Check sheet for the drawn part. Datum: minimum x, y, z corner. Units: mm. A direction names the side the tool comes from. Give positions to 0.01 mm unless a question says otherwise; leave off trailing zeros. Loops run counter-clockwise (first coordinate to the right, second up) from the corner with the lowest first, then second, coordinate; pieces in that order, holes last. Notation, with made-up numbers: (-10.75, -2.5) - (22.25, -2.5) arc R26 cw to (22.25, 19.5) - close; hole circle Ø8 at (84, 73.25). An arc over 180 degrees is marked (long way). Answer in a Markdown table with one row per item.
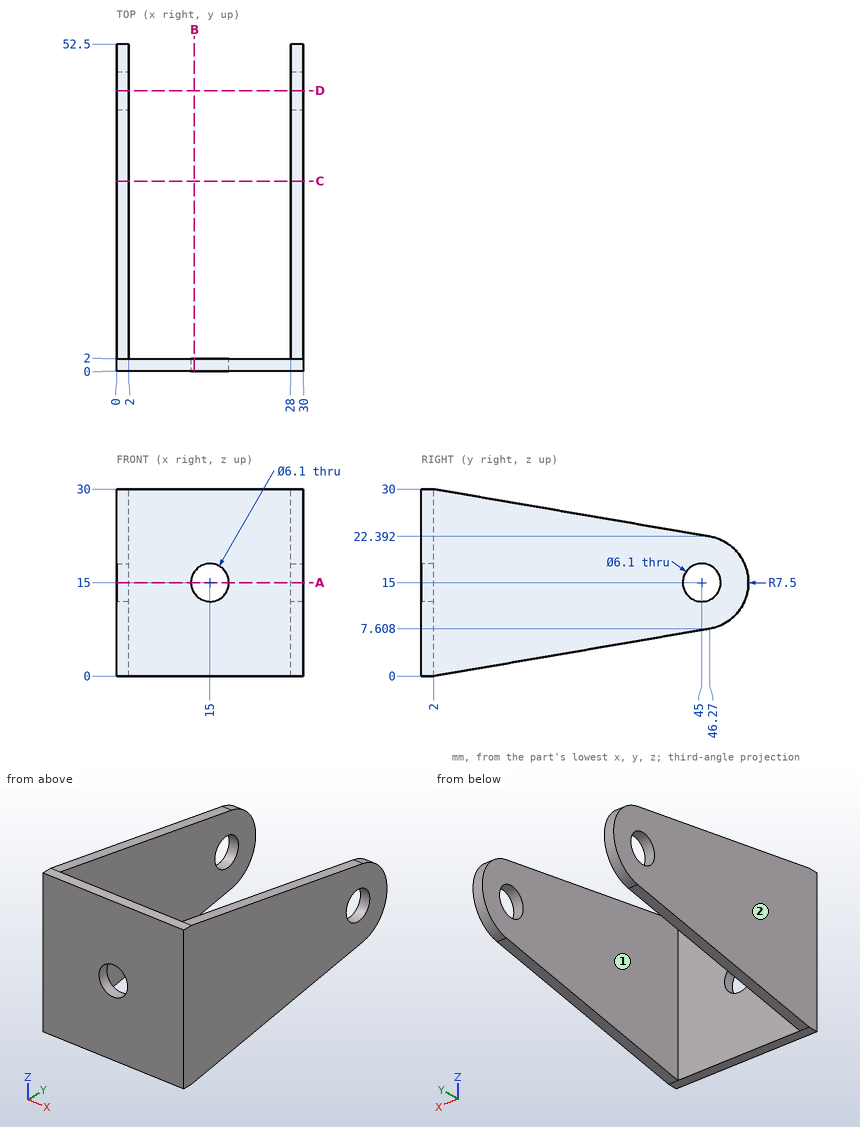
Q1. Tool access check on the marked faces 1 and 2. Record the directions out of +Z, -Z, +X, -X, +Y, -Y that give a thin tool (end or side, any length) a straight path to the whole face; none if there is none.
Completed:
| item | result |
|---|---|
| face 1 | +Z, -Z, +Y |
| face 2 | +Z, -Z, -X, +Y, -Y |
Q2. Go/stop test with a flat-tipped pin: P1, Ø8, axis at x = 14.5, z = 8.5, coming from the +Y side. Record where the tip stops, or that it passes through.
Completed:
| item | result |
|---|---|
| P1 | y = 2 |
Q3. Sectioned sample at A-A (z = 15). Record the cut outline in (x, y).
Completed:
| item | result |
|---|---|
| outline | (0, 0) - (11.95, 0) - (11.95, 2) - (2, 2) - (2, 41.95) - (0, 41.95) - close; (0, 48.05) - (2, 48.05) - (2, 52.5) - (0, 52.5) - close; (18.05, 0) - (30, 0) - (30, 41.95) - (28, 41.95) - (28, 2) - (18.05, 2) - close; (28, 48.05) - (30, 48.05) - (30, 52.5) - (28, 52.5) - close |
Q4. Sectioned sample at B-B (x = 12.5). Record the cut outline in (y, z).
Completed:
| item | result |
|---|---|
| outline | (0, 0) - (2, 0) - (2, 13.25) - (0, 13.25) - close; (0, 16.75) - (2, 16.75) - (2, 30) - (0, 30) - close |
Q5. Sectioned sample at C-C (y = 30.5). Record the cut outline in (x, z).
Completed:
| item | result |
|---|---|
| outline | (0, 4.9) - (2, 4.9) - (2, 25.1) - (0, 25.1) - close; (28, 4.9) - (30, 4.9) - (30, 25.1) - (28, 25.1) - close |
Q6. Sectioned sample at D-D (y = 45). Record the cut outline in (x, z).
Completed:
| item | result |
|---|---|
| outline | (0, 7.39) - (2, 7.39) - (2, 11.95) - (0, 11.95) - close; (0, 18.05) - (2, 18.05) - (2, 22.61) - (0, 22.61) - close; (28, 7.39) - (30, 7.39) - (30, 11.95) - (28, 11.95) - close; (28, 18.05) - (30, 18.05) - (30, 22.61) - (28, 22.61) - close |
Q7. Thickness scan on line 1 (X direction, y = 8, z = 11); line 2 (Z direction, x = 15, y = 1.25); line 3 (Y direction, x = 1.55, z = 15). Record the ranges inside material, lowest first.
Completed:
| item | result |
|---|---|
| line 1 | 0 to 2, 28 to 30 |
| line 2 | 0 to 11.95, 18.05 to 30 |
| line 3 | 0 to 41.95, 48.05 to 52.5 |
